from build123d import *

# Parameters (mm, degrees)
SKETCH1_W           = 11.8745
SKETCH1_H           = 9.9187
BOSS_EXTRUDE1_DEPTH = 25.2984
SKETCH2_R           = 2.0066
BOSS_EXTRUDE2_DEPTH = 0.762
SKETCH3_R           = 1.5113
BOSS_EXTRUDE3_DEPTH = 9.0932
CUT_EXTRUDE1_DEPTH  = 5.9436


with BuildPart() as part:
    # Sketch1 → Boss-Extrude1 (new body)
    with BuildSketch(Plane.XY):
        Rectangle(SKETCH1_W, SKETCH1_H)
    extrude(amount=-BOSS_EXTRUDE1_DEPTH)

    # Sketch2 → Boss-Extrude2 (add)
    with BuildSketch(Plane.XY):
        Circle(SKETCH2_R)
    extrude(amount=BOSS_EXTRUDE2_DEPTH)

    # Sketch3 → Boss-Extrude3 (add)
    with BuildSketch(Plane.XY.offset(0.762)):
        Circle(SKETCH3_R)
    extrude(amount=BOSS_EXTRUDE3_DEPTH)

    # Sketch4 → Cut-Extrude1 (cut)
    with BuildSketch(Plane.XY.offset(9.8552)):
        Polygon((-31.544055033, 0.9652), (-1.667569456, 0.9652), (2.041996645, 0.9652), (31.918482222, 0.9652), (31.918482222, 60.718171154), (-31.544055033, 60.718171154), align=None)
    extrude(amount=-CUT_EXTRUDE1_DEPTH, mode=Mode.SUBTRACT)


solid = part.part
Here's how the part is built. I have some questions about the finished solid (model axes, mm). A direction names the side the tool comes from. Give positions to 0.01 mm unless a question says otherwise; leave off trailing zeros. Order: outer loops, then holes, each group sorted by start corner. A loop starts at its lowest first (then second) coordinate and runs counter-clockwise, first axis right, second up. Notation, with made-up numbers: (64.5, 75.5) -> (84.5, 75.5) arc R35 ccw to (84.5, 109.5) -> close; hole circle Ø1 at (11.25, 51.25). An arc over 180 degrees is marked (long way). Use a Markdown table: item, result. Add a question column.
Item 1: I need wall thicknesses on line 1 (Z direction, x = 2.25, y = 0.25); line 2 (Y direction, x = -1, z = 5.5). Which ranges of each line are inside material? Lowest first, please.
Item 2: Imagine slicing it at B-B on x = 0. Please give me the cut outline in (y, z).
Item 3: Imagine slicing it at D-D on y = 3.5. Please give me the cut outline in (x, z), plus the area to 3 significant figures.
Item 4: Imagine slicing it at A-A on y = 0. Please give me the cut outline in (x, z), plus the area to 3 significant figures.
Item 5: For faces 1 (the face through (-0.1, 2.3, 0)), 2 (the face through (0, 4.959, -12)), 3 (the face through (0, 0.965, 7)), which set-ups out of +Z, -Z, +X, -X, +Y, -Y let a thin tool reach every point of the face, with its end or its side?
Item 6: Will these pins go through, and if not, where does the flat tip stop? pin 1 (2.5 mm diameter, centred on x = 0.5, z = 7, fed in from +Y); pin 2 (2 mm diameter, centred on x = -1.5, y = 4, fed in from +Z); pin 3 (1.5 mm diameter, centred on x = -4, z = 6.5, fed in from -Y); pin 4 (0.6 mm diameter, centred on x = 0, y = 1.5, fed in from +Z).
Item 7: Imagine slicing it at C-C on z = 5. Please give me the cut outline in (x, y).
Data:
| question | item | result |
|---|---|---|
| 1 | line 1 | z = -25.3 to 0 |
| 1 | line 2 | y = -1.13 to 0.97 |
| 2 | outline | (-4.96, -25.3) -> (4.96, -25.3) -> (4.96, 0) -> (2.01, 0) -> (2.01, 0.76) -> (1.51, 0.76) -> (1.51, 3.91) -> (0.97, 3.91) -> (0.97, 9.86) -> (-1.51, 9.86) -> (-1.51, 0.76) -> (-2.01, 0.76) -> (-2.01, 0) -> (-4.96, 0) -> close |
| 3 | outline | (-5.94, -25.3) -> (5.94, -25.3) -> (5.94, 0) -> (-5.94, 0) -> close |
| 3 | area | 300 mm² |
| 4 | outline | (-5.94, -25.3) -> (5.94, -25.3) -> (5.94, 0) -> (2.01, 0) -> (2.01, 0.76) -> (1.51, 0.76) -> (1.51, 9.86) -> (-1.51, 9.86) -> (-1.51, 0.76) -> (-2.01, 0.76) -> (-2.01, 0) -> (-5.94, 0) -> close |
| 4 | area | 331 mm² |
| 5 | face 1 | +Z |
| 5 | face 2 | +Z, -Z, +X, -X, +Y |
| 5 | face 3 | +Z, +X, -X, +Y |
| 6 | pin 1 | stops at y = 0.97 |
| 6 | pin 2 | stops at z = 0 |
| 6 | pin 3 | passes through |
| 6 | pin 4 | stops at z = 3.91 |
| 7 | outline | (-1.16, 0.97) arc R1.51 ccw (long way) to (1.16, 0.97) -> close |
